Autodesk Inventor part; units mm, degrees
ref_plane "YZ Plane" through (0, 0, 0) normal (1, 0, 0) x (0, 1, 0)
ref_plane "XZ Plane" through (0, 0, 0) normal (0, 1, 0) x (-1, 0, 0)
ref_plane "XY Plane" through (0, 0, 0) normal (0, 0, 1) x (1, 0, 0)
sketch "スケッチ1" plane through (0, 0, 0) normal (0, 0, 1) x (1, 0, 0)
  circle A0 centre (0, 0) radius 2
  dimension "d0" = 4
extrude "押し出し1" add sketch "スケッチ1" along normal blind 6
sketch "スケッチ2" plane through (0, 0, 6) normal (0, 0, 1) x (1, 0, 0)
  circle A0 centre (0, 0) radius 2
  circle A1 centre (0, 0) radius 4
  dimension "d3" = 8
extrude "押し出し2" add sketch "スケッチ2" along normal blind 2.3 contours A0 | A1
thread "ねじ1"
chamfer "面取り1" distance 2 angle 45 1 edges at (-4, 0, 6)
sketch "スケッチ4" plane through (0, 0, 0) normal (0, 0, -1) x (-1, 0, 0)
  circle A0 centre (0, 0) radius 2
extrude "押し出し4" add sketch "スケッチ4" along normal blind 1.7
properties part number "SB　M4 10mm 皿ネジ" material "Stainless Steel, 440C"
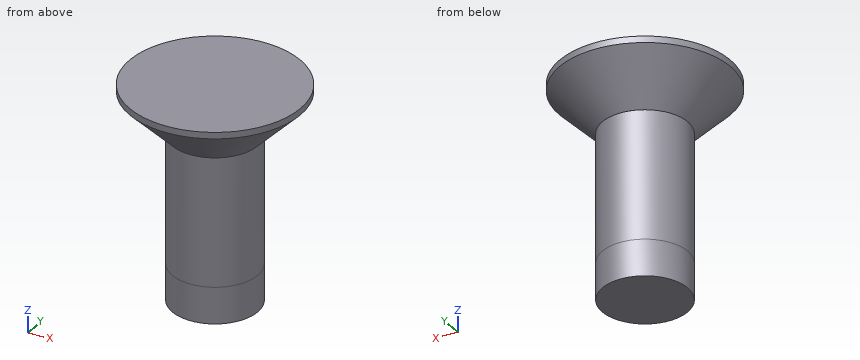
Work out the finished part from the listing and answer in its coordinate system (mm). Coordinates: 2 decimals unless noted, no trailing zeros. Write each loop counter-clockwise with the first axis right and the second up, starting at its lowest first coordinate (ties: lowest second). Pieces come first, ordered by that corner, then holes. Notation, with made-up numbers: M 23.25,-14 L 61.25,-14 A15 cw 61.25,-1 Z; hole C -12,35 d2. An arc over 180 degrees is marked long. Write item = value, one per line.
1. The part is cut by section C-C (z = 3.5). Determine the outline of the cut face in (x, y), then the cut area to 3 significant figures.
Solution:
outline = C 0,0 d4
area = 12.6 mm2
2. Flat-ended cylindrical pins translate along their axes: pin 1 (3 mm diameter, centred on x = 1.5, z = 2.5, fed in from +Y); pin 2 (1 mm diameter, centred on x = 1, y = -2.5, fed in from -Z); pin 3 (3 mm diameter, centred on x = 2.5, y = 1, fed in from -Z). Find the tip coordinate at first contact, or state that the pin passes through.
Solution:
pin_1 = 2
pin_2 = 6.19
pin_3 = -1.7
3. Straight lines are drawn through the part: line 1 (Z direction, x = 3.75, y = -0.5); line 2 (Z direction, x = 3, y = 0.75); line 3 (X direction, y = -0.5, z = 3). For each, find the intervals that lie inside material, in ascending order. Write a range as from..to.
Solution:
line_1 = 7.78..8.3
line_2 = 7.09..8.3
line_3 = -1.94..1.94
4. The part is cut by section D-D (z = 7.75). Determine the outline of the cut face in (x, y), then the cut area to 3 significant figures.
Solution:
outline = C 0,0 d7.5
area = 44.2 mm2
